Build history of the part. All positions in model axes, mm. Give positions to 0.01 mm unless a question says otherwise; leave off trailing zeros. Order: outer loops, then holes, each group sorted by start corner. A loop starts at its lowest first (then second) coordinate and runs counter-clockwise, first axis right, second up. Notation, with made-up numbers: (79, -17) - (99, -17) arc R21 cw to (99, 22) - close; hole circle Ø9 at (-0.75, 36.25). An arc over 180 degrees is marked (long way). Use a Markdown table: item, result. Add a question column.
(1) Wall check: line 1 (Y direction, x = -114.5, z = 0.3); line 2 (X direction, y = -3, z = 4.8); line 3 (Y direction, x = 29.5, z = 1.9). Give the ranges that are in metal, low to high.
(2) Flat gauge pins, fed straight in: pin 1 (1.5 mm diameter, centred on x = -115, z = 2, fed in from +Y); pin 2 (2.5 mm diameter, centred on y = -26, z = 2.5, fed in from +X); pin 3 (1.5 mm diameter, centred on x = 134, z = 2, fed in from +Y). Where does each tip first touch, or does it go through?
(3) Slice it at D-D (y = 82). Write the cut outline in (x, z).
(4) Slice it at C-C (x = -34.5). Write the cut outline in (y, z).
(5) Slice it at A-A (y = 23). Write the cut outline in (x, z), then the cut area to 4 significant figures.
(6) Slice it at B-B (z = 4.2). Count the separate pieces of the cut face and the enclosed holes in it, then the cut area to 3 significant figures.
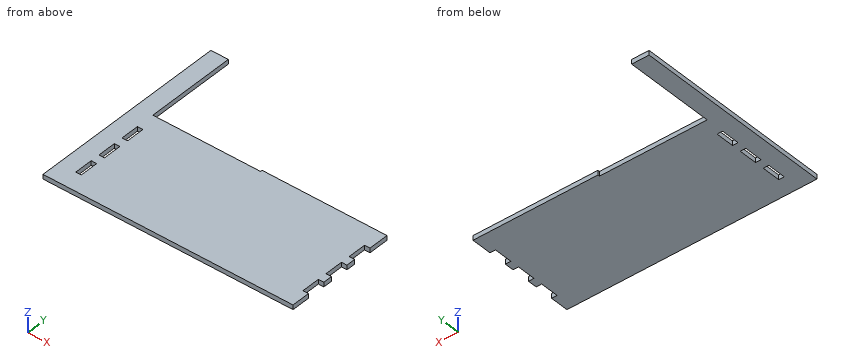
from build123d import *

# Parameters (mm, degrees)
SKETCH1_W           = 273
SKETCH1_H           = 122
BOSS_EXTRUDE1_DEPTH = 5
SKETCH2_W           = 19
SKETCH2_H           = 96
BOSS_EXTRUDE2_DEPTH = 5
SKETCH3_W           = 6
SKETCH3_H           = 20
CUT_EXTRUDE1_DEPTH  = 6
SKETCH6_W           = 117.5
SKETCH6_H           = 2
CUT_EXTRUDE3_DEPTH  = 6


with BuildPart() as part:
    # Sketch1 → Boss-Extrude1 (new body)
    with BuildSketch(Plane.XY):
        Rectangle(SKETCH1_W, SKETCH1_H)
    extrude(amount=BOSS_EXTRUDE1_DEPTH)

    # Sketch2 → Boss-Extrude2 (add)
    with BuildSketch(Plane.XY.offset(5)):
        with Locations((-127, 109)):
            Rectangle(SKETCH2_W, SKETCH2_H)
    extrude(amount=-BOSS_EXTRUDE2_DEPTH)

    # Sketch3 → Cut-Extrude1 (cut)
    with BuildSketch(Plane.XY.offset(5)):
        with Locations((-114.5, 29)):
            Rectangle(SKETCH3_W, SKETCH3_H)
        with Locations((-114.5, -1)):
            Rectangle(SKETCH3_W, SKETCH3_H)
        with Locations((-114.5, -31)):
            Rectangle(SKETCH3_W, SKETCH3_H)
        with Locations((133.5, 29)):
            Rectangle(SKETCH3_W, SKETCH3_H)
        with Locations((133.5, -1)):
            Rectangle(SKETCH3_W, SKETCH3_H)
        with Locations((133.5, -31)):
            Rectangle(SKETCH3_W, SKETCH3_H)
    extrude(amount=-CUT_EXTRUDE1_DEPTH, mode=Mode.SUBTRACT)

    # Sketch6 → Cut-Extrude3 (cut)
    with BuildSketch(Plane.XY.offset(5)):
        with Locations((-58.75, 60)):
            Rectangle(SKETCH6_W, SKETCH6_H)
    extrude(amount=-CUT_EXTRUDE3_DEPTH, mode=Mode.SUBTRACT)


solid = part.part
Solution:
| question | item | result |
|---|---|---|
| 1 | line 1 | -61 to -41, -21 to -11, 9 to 19, 39 to 59 |
| 1 | line 2 | -136.5 to -117.5, -111.5 to 130.5 |
| 1 | line 3 | -61 to 61 |
| 2 | pin 1 | y = 59 |
| 2 | pin 2 | x = 130.5 |
| 2 | pin 3 | y = 61 |
| 3 | outline | (-136.5, 0) - (-117.5, 0) - (-117.5, 5) - (-136.5, 5) - close |
| 4 | outline | (-61, 0) - (59, 0) - (59, 5) - (-61, 5) - close |
| 5 | outline | (-136.5, 0) - (-117.5, 0) - (-117.5, 5) - (-136.5, 5) - close; (-111.5, 0) - (130.5, 0) - (130.5, 5) - (-111.5, 5) - close |
| 5 | area | 1,305 mm2 |
| 6 | separate pieces | 1 |
| 6 | enclosed holes | 3 |
| 6 | area | 34,200 mm2 |
